from build123d import *

# Parameters (mm, degrees)
SKETCH_1_W        = 5
SKETCH_1_H        = 8
SKETCH_1_R        = 1.5
EXTRUDE_1_DEPTH   = 2
EXTRUDE_1_2_DEPTH = 2
EXTRUDE_START     = 2
SKETCH_1_6_W      = 5
SKETCH_1_6_H      = 3
EXTRUDE_2_DEPTH   = 16
SKETCH_2_W        = 5
SKETCH_2_H        = 3
EXTRUDE_3_DEPTH   = 43.4


with BuildPart() as part:
    # Sketch 1 → Extrude 1 (new body)
    with BuildSketch(Plane(origin=(0, 0, 0), x_dir=(1, 0, 0), z_dir=(0, 1, 0))):
        with Locations((2.5, -4)):
            Rectangle(SKETCH_1_W, SKETCH_1_H)
        with Locations(Location((2.5, -2.5, 0), (0, 0, 270))):
            Circle(SKETCH_1_R, mode=Mode.SUBTRACT)
    extrude(amount=EXTRUDE_1_DEPTH)



with BuildPart() as body_2:
    # Sketch 1 → Extrude 1 2 (new body)
    with BuildSketch(Plane(origin=(0, 0, 0), x_dir=(1, 0, 0), z_dir=(0, 1, 0))):
        with Locations((2.5, -49.4)):
            Rectangle(SKETCH_1_W, SKETCH_1_H)
        with Locations(Location((2.5, -50.9, 0), (0, 0, 270))):
            Circle(SKETCH_1_R, mode=Mode.SUBTRACT)
    extrude(amount=EXTRUDE_1_2_DEPTH)


with BuildPart() as part_1:
    add(part.part)

    add(body_2.part)  # Extrude 2 merges body 2
    # Sketch 1_6 → Extrude 2 (add)
    with BuildSketch(Plane(origin=(0, 0, 0), x_dir=(1, 0, 0), z_dir=(0, 1, 0)).offset(EXTRUDE_START)):
        with Locations((2.5, -46.9)):
            Rectangle(SKETCH_1_6_W, SKETCH_1_6_H)
        with Locations((2.5, -6.5)):
            Rectangle(SKETCH_1_6_W, SKETCH_1_6_H)
    extrude(amount=-EXTRUDE_2_DEPTH)

    # Sketch 2 → Extrude 3 (add)
    with BuildSketch(Plane.XY.offset(48.4)):
        with Locations((2.5, -15.5)):
            Rectangle(SKETCH_2_W, SKETCH_2_H)
    extrude(amount=-EXTRUDE_3_DEPTH)


solid = part_1.part
Could you check a few things on this model? Use its own coordinates, in mm. A direction names the side the tool comes from. Give positions to 0.01 mm unless a question says otherwise; leave off trailing zeros. Order: outer loops, then holes, each group sorted by start corner. A loop starts at its lowest first (then second) coordinate and runs counter-clockwise, first axis right, second up. Notation, with made-up numbers: (8, 31) -> (37, 31) arc R8 ccw to (37, 41) -> close; hole circle Ø9 at (83, 84). An arc over 180 degrees is marked (long way). Answer in a Markdown table with one row per item. Add a question column.
Item 1: For faces 1 (the flat face through (2, -6, 45.4)), 2 (the flat face through (1, 0, 1)), 3 (the flat face through (2, -8, 48.4)), which set-ups out of +Z, -Z, +X, -X, +Y, -Y let a thin tool reach every point of the face, with its end or its side?
Item 2: Imagine slicing it at C-C (x = 2.5). List the corners of the cut face in (y, z) for me.
Item 3: Imagine slicing it at D-D (z = 29). List the corners of the cut face in (x, y) for me, and give its area (3 significant figures).
Item 4: Imagine slicing it at B-B (y = -8.5). List the corners of the cut face in (x, z) for me.
Item 5: Please list where these lines run through material, in increasing order: probe 1 along X at (y, z) = (1.25, 2.5); probe 2 along Z at (x, y) = (0.4, -7.25); probe 3 along Y at (x, z) = (0.3, 17.5).
Item 6: I'm going to push flat-ended pins straight in: P1, Ø8, axis at y = -7.5, z = 34.5, coming from the +X side; P2, Ø1, axis at x = 3, y = -3, coming from the -Z side; P3, Ø1.5, axis at x = 2, y = -8, coming from the +Z side; P4, Ø1.5, axis at x = 3, z = 3.5, coming from the -Y side. Where does each tip first touch, or does it pass through?
Item 7: Imagine slicing it at A-A (z = 2.5). List the corners of the cut face in (x, y) for me.
Item 8: We'd pull the mould along Z, two halves only. Please class faces 4 (the flat face through (2, -8, 5)), 5 (the flat face through (5, -15, 25)), 6 (the flat face through (2, -6, 8)): pulls with the +Z half, pulls with the -Z half, needs draft (parallel to the pull), parting line crosses it, or undercut.
Result:
| question | item | result |
|---|---|---|
| 1 | face 1 | +X, -X, +Y |
| 1 | face 2 | -Z, +X, -X, -Y |
| 1 | face 3 | +Z, +X, -X, -Y |
| 2 | outline | (-17, 5) -> (0, 5) -> (0, 4) -> (2, 4) -> (2, 8) -> (-14, 8) -> (-14, 45.4) -> (2, 45.4) -> (2, 49.4) -> (0, 49.4) -> (0, 48.4) -> (-17, 48.4) -> close; (0, 0) -> (2, 0) -> (2, 1) -> (0, 1) -> close; (0, 52.4) -> (2, 52.4) -> (2, 53.4) -> (0, 53.4) -> close |
| 3 | outline | (0, -17) -> (5, -17) -> (5, -14) -> (0, -14) -> close |
| 3 | area | 15.0 mm2 |
| 4 | outline | (0, 5) -> (5, 5) -> (5, 8) -> (0, 8) -> close; (0, 45.4) -> (5, 45.4) -> (5, 48.4) -> (0, 48.4) -> close |
| 5 | probe 1 | 0 to 1, 4 to 5 |
| 5 | probe 2 | 5 to 8, 45.4 to 48.4 |
| 5 | probe 3 | -17 to -14 |
| 6 | P1 | through |
| 6 | P2 | z = 5 |
| 6 | P3 | z = 48.4 |
| 6 | P4 | y = 0 |
| 7 | outline | (0, 0) -> (1, 0) -> (1, 2) -> (0, 2) -> close; (4, 0) -> (5, 0) -> (5, 2) -> (4, 2) -> close |
| 8 | face 4 | pulls with the -Z half |
| 8 | face 5 | needs draft |
| 8 | face 6 | undercut |
